Source: CAD feature listing. Evaluate the final solid. Frame: model axes, mm. Give positions to 0.01 mm unless a question says otherwise; leave off trailing zeros. Loops run counter-clockwise (first coordinate to the right, second up) from the corner with the lowest first, then second, coordinate; pieces in that order, holes last. Notation, with made-up numbers: M 45.5,33.5 L 101.5,33.5 A11 cw 101.5,38.5 Z; hole C -28.75,6 d11. An arc over 180 degrees is marked long. Answer in a Markdown table with one row per item.
Autodesk Inventor part; units mm, degrees
ref_plane "YZ Plane" through (0, 0, 0) normal (1, 0, 0) x (0, 1, 0)
ref_plane "XZ Plane" through (0, 0, 0) normal (0, 1, 0) x (-1, 0, 0)
ref_plane "XY Plane" through (0, 0, 0) normal (0, 0, 1) x (1, 0, 0)
sketch "スケッチ1 outline for 押し出し1" plane through (0, 0, 0) normal (0, 0, 1) x (1, 0, 0)
  line L0 (-1089.396157, 354.695803) -> (-1151.82556, 342.195803)
  line L1 (-1089.396157, 274.695803) -> (-1089.396157, 354.695803)
  line L2 (-1151.82556, 342.195803) -> (-1151.82556, 309.195803)
  line L3 (-1109.396157, 274.695803) -> (-1089.396157, 274.695803)
  line L4 (-1151.82556, 309.195803) -> (-1109.396157, 274.695803)
  circle A0 centre (-1099.396157, 282.695803) radius 4.5
  circle A1 centre (-1146.82556, 314.695803) radius 2.75
  circle A2 centre (-1146.82556, 336.695803) radius 2.75
  circle A3 centre (-1114.82556, 314.695803) radius 2.75
  circle A4 centre (-1114.82556, 336.695803) radius 2.75
  circle A5 centre (-1099.396157, 346.695803) radius 4.5
extrude "押し出し1" add sketch "スケッチ1 outline for 押し出し1" along normal blind 14.016552
1) Section C-C, the plane y = 345. Return loops of the section in (x, z), then the cut area to 3 significant figures.
Reply:
| item | result |
|---|---|
| outline | M -1137.82,0 L -1103.56,0 L -1103.56,14.02 L -1137.82,14.02 Z; M -1095.23,0 L -1089.4,0 L -1089.4,14.02 L -1095.23,14.02 Z |
| area | 562 mm² |
2) Section D-D, the plane x = -1146.5. Return loops of the section in (y, z), then the cut area to 3 significant figures.
Reply:
| item | result |
|---|---|
| outline | M 304.87,0 L 311.97,0 L 311.97,14.02 L 304.87,14.02 Z; M 317.43,0 L 333.97,0 L 333.97,14.02 L 317.43,14.02 Z; M 339.43,0 L 343.26,0 L 343.26,14.02 L 339.43,14.02 Z |
| area | 385 mm² |
3) Section B-B, the plane z = 13. Return loops of the section in (x, y), then the cut area to 3 significant figures.
Reply:
| item | result |
|---|---|
| outline | M -1151.83,309.2 L -1109.4,274.7 L -1089.4,274.7 L -1089.4,354.7 L -1151.83,342.2 Z; hole C -1146.83,314.7 d5.5; hole C -1146.83,336.7 d5.5; hole C -1114.83,314.7 d5.5; hole C -1114.83,336.7 d5.5; hole C -1099.4,282.7 d9; hole C -1099.4,346.7 d9 |
| area | 3,650 mm² |
4) Pull-direction query (Y, two-part tool) for faces 1 (the cylindrical face through (-1103, 280, 7)), 2 (the flat face through (-1121, 315, 14.017)), 3 (the cylindrical face through (-1144.285, 315.749, 6.91)), 4 (the flat face through (-1130.91, 292.19, 6.91)); classes: released by +Y, released by -Y, zero draft, split by the parting line, or undercut.
Reply:
| item | result |
|---|---|
| face 1 | undercut |
| face 2 | zero draft |
| face 3 | undercut |
| face 4 | released by -Y |
5) Material intervals for L1, parallel to X at y = 334.5, z = 13.25; L2, parallel to Y at x = -1102, z = 3; L3, parallel to X at y = 339, z = 2.75, sorted ascending.
Reply:
| item | result |
|---|---|
| L1 | x = -1151.83 to -1148.48, -1145.17 to -1116.48, -1113.17 to -1089.4 |
| L2 | y = 274.7 to 279.03, 286.37 to 343.03, 350.37 to 352.17 |
| L3 | x = -1151.83 to -1148.33, -1145.32 to -1116.33, -1113.32 to -1089.4 |
6) Pin query (flat end, axial travel): pin 1 Ø5 at (x, y) = (-1114.83, 336.7) entering from +Z; pin 2 Ø3 at (x, z) = (-1141, 11.5) entering from -Y; pin 3 Ø5 at (x, z) = (-1113, 11) entering from +Y. Return the tip coordinate at first contact, or that it passes through.
Reply:
| item | result |
|---|---|
| pin 1 | passes through |
| pin 2 | stops at y = 299.17 |
| pin 3 | stops at y = 350.47 |
7) Section A-A, the plane x = -1099. Return loops of the section in (y, z), then the cut area to 3 significant figures.
Reply:
| item | result |
|---|---|
| outline | M 274.7,0 L 278.21,0 L 278.21,14.02 L 274.7,14.02 Z; M 287.18,0 L 342.21,0 L 342.21,14.02 L 287.18,14.02 Z; M 351.18,0 L 352.77,0 L 352.77,14.02 L 351.18,14.02 Z |
| area | 843 mm² |
